Can you work these out from the model? Positions are in its coordinate system, mm. A direction names the side the tool comes from. Coordinates: 2 decimals unless noted, no trailing zeros. Order: outer loops, then holes, each group sorted by start corner. A loop starts at its lowest first (then second) coordinate and runs counter-clockwise, first axis right, second up. Notation, with made-up numbers: (3.25, 53) -> (60.25, 53) arc R18 cw to (60.25, 86) -> close; hole circle Ø6 at (5, 85.25). An arc over 180 degrees is marked (long way). Answer in a Markdown table with one row per item. Add a question column.
1. Imagine slicing it at B-B on x = 21. Write out the boundary of the cut face in (y, z).
2. If I drill on line 1 along Y through (x, z) = (28, 4.5); line 2 along X through (y, z) = (-6, 9); line 3 along Z through (x, y) = (-12.5, -20.5), over which ranges is the centre line in solid material (lowest first)? Write a range as [from, to].
3. Will these pins go through, and if not, where does the flat tip stop? pin 1 (3 mm diameter, centred on x = -16.25, y = -19.88, fed in from +Z); pin 2 (2.5 mm diameter, centred on y = -6.5, z = 8.5, fed in from +X); pin 3 (2.5 mm diameter, centred on x = 5, z = 5.5, fed in from +Y).
4. Imagine slicing it at A-A on y = -9. Write out the boundary of the cut face in (x, z).
5. On a 3-axis mill with a long thin cutter (end or side, diameter ignored), from which of +Z, -Z, +X, -X, +Y, -Y can I reach the whole of each face in a straight line? I mean faces 1 (the face through (-14.895, -5, 6)), 2 (the face through (21, 8.525, 6)), 3 (the face through (21, -17.475, 6)). Say none if no direction works.
6. We'd pull the mould along X, two halves only. Please class faces 4 (the face through (-15, 11, 1)), 5 (the face through (61.255, -5, 1)), 6 (the face through (21, 13.625, 1)): pulls with the +X half, pulls with the -X half, needs draft (parallel to the pull), parting line crosses it, or undercut.
7. Imagine slicing it at C-C on z = 2.75. Write out the boundary of the cut face in (x, y), plus the area to 3 significant figures.
from build123d import *

# Parameters (mm, degrees)
SKETCH_1_W          = 80
SKETCH_1_H          = 36
EXTRUDE_1_DEPTH     = 2
SKETCH_2_W          = 72
SKETCH_2_H          = 26
EXTRUDE_2_DEPTH     = 9
SKETCH_3_R          = 1.25
CUT_EXTRUDE_1_DEPTH = 66.831593266


with BuildPart() as part:
    # Эскиз1 → Бобышка-Вытянуть1 (new body)
    with BuildSketch(Plane.XY):
        with Locations((21.254780468, -4.375221601)):
            Rectangle(SKETCH_1_W, SKETCH_1_H)
    extrude(amount=EXTRUDE_1_DEPTH)

    # Эскиз2 → Бобышка-Вытянуть2 (add)
    with BuildSketch(Plane.XY.offset(2)):
        with Locations((21.104780468, -4.475221601)):
            Rectangle(SKETCH_2_W, SKETCH_2_H)
    extrude(amount=EXTRUDE_2_DEPTH)

    # Эскиз3 → Вырез-Вытянуть1 (cut, through all)
    with BuildSketch(Plane.XY.offset(2)):
        with Locations((-16.245219532, 11.124778399)):
            Circle(SKETCH_3_R)
        with Locations((58.754780468, 11.124778399)):
            Circle(SKETCH_3_R)
        with Locations((58.754780468, -19.875221601)):
            Circle(SKETCH_3_R)
        with Locations((-16.245219532, -19.875221601)):
            Circle(SKETCH_3_R)
    extrude(amount=-CUT_EXTRUDE_1_DEPTH, mode=Mode.SUBTRACT)


solid = part.part
Answers follow:
| question | item | result |
|---|---|---|
| 1 | outline | (-22.38, 0) -> (13.62, 0) -> (13.62, 2) -> (8.52, 2) -> (8.52, 11) -> (-17.48, 11) -> (-17.48, 2) -> (-22.38, 2) -> close |
| 2 | line 1 | y = [-17.48, 8.52] |
| 2 | line 2 | x = [-14.9, 57.1] |
| 2 | line 3 | z = [0, 2] |
| 3 | pin 1 | stops at z = 2 |
| 3 | pin 2 | stops at x = 57.1 |
| 3 | pin 3 | stops at y = 8.52 |
| 4 | outline | (-18.75, 0) -> (61.25, 0) -> (61.25, 2) -> (57.1, 2) -> (57.1, 11) -> (-14.9, 11) -> (-14.9, 2) -> (-18.75, 2) -> close |
| 5 | face 1 | +Z, -X, +Y, -Y |
| 5 | face 2 | +Z, +X, -X, +Y |
| 5 | face 3 | +Z, +X, -X, -Y |
| 6 | face 4 | undercut |
| 6 | face 5 | pulls with the +X half |
| 6 | face 6 | needs draft |
| 7 | outline | (-14.9, -17.48) -> (57.1, -17.48) -> (57.1, 8.52) -> (-14.9, 8.52) -> close |
| 7 | area | 1,870 mm² |
